Check sheet for the modelled part. Datum: model origin and axes. Units: mm. A direction names the side the tool comes from. Round coordinates to 2 decimals unless told otherwise and drop trailing zeros. Loops run counter-clockwise (first coordinate to the right, second up) from the corner with the lowest first, then second, coordinate; pieces in that order, holes last. Notation, with made-up numbers: M 77.5,24.25 L 124.5,24.25 A26 cw 124.5,51.25 Z; hole C 24.5,72 d11. An arc over 180 degrees is marked long. Write item = value, one per line. Start each with the question number.
(1) Cross-section at B-B on x = -24.5. Record the boundary of the cut face in (y, z).
(2) Cross-section at C-C on x = 7. Record the boundary of the cut face in (y, z), plus the area to 3 significant figures.
(3) Set-up check for faces 1 (the face through (-20, 12, 0)), 2 (the face through (20, 32, 0)), 3 (the face through (20, 12, 0)), 4 (the face through (-20, 30, 0)): record each of +Z, -Z, +X, -X, +Y, -Y from which the full face is reachable in a straight line by a thin tool's end or side.
(4) Mould release check, pull along X, two halves, no side actions. Record for faces 5 (the face through (0, 0, 0)), 6 (the face through (7, 37.5, 0)), 7 (the face through (-12.112, 35.472, -0.14)): pulls with the +X half, pulls with the -X half, needs draft (parallel to the pull), parting line crosses it, or undercut.
(5) Cross-section at D-D on z = 0. Record the boundary of the cut face in (x, y).
(6) Go/stop test with flat-tipped pins: P1, Ø9, axis at x = 25.5, z = 1, coming from the -Y side; P2, Ø10, axis at y = 13, z = -7, coming from the +X side; P3, Ø2.5, axis at x = -24.5, z = -1, coming from the +Y side. Record where each tip stops, or that it passes through.
(7) Cross-section at A-A on z = 5. Record the boundary of the cut face in (x, y), plus the area to 3 significant figures.
(8) Scan lines: L1, parallel to Z at x = 24.5, y = 26.6; L2, parallel to X at y = 26.2, z = 5; L3, parallel to Z at x = 7, y = 38. Record each from-to range of solid material in increasing order. Write a range as from..to.
Autodesk Inventor part; units mm, degrees
ref_plane "Work Plane1" through (0, 24.7, 0) normal (0, -1, 0) x (1, 0, 0)
ref_plane "YZ Plane" through (0, 0, 0) normal (1, 0, 0) x (0, 1, 0)
ref_plane "XZ Plane" through (0, 0, 0) normal (0, 1, 0) x (-1, 0, 0)
sketch "Sketch1" plane through (0, 0, 0) normal (0, 1, 0) x (-1, 0, 0)
  line L0 (20, 10) -> (-20, 10)
  line L1 (-20, 10) -> (-20, -10)
  line L2 (-20, -10) -> (20, -10)
  line L3 (20, -10) -> (20, 10)
  line L4 (20, 10) -> (-20, -10) construction
  line L5 (-20, 10) -> (20, -10) construction
  point P0 (0, 0)
  dimension "d0" = 40
  dimension "d1" = 20
extrude "Extrusion1" add sketch "Sketch1" along normal blind 37.5
ref_plane "Work Plane1" through (0, 24.7, 0) normal (0, -1, 0) x (1, 0, 0)
sketch "Sketch2" plane through (0, 24.7, 0) normal (0, -1, 0) x (1, 0, 0)
  line L0 (-28, 10) -> (28, 10)
  line L1 (28, 10) -> (28, -10)
  line L2 (28, -10) -> (-28, -10)
  line L3 (-28, -10) -> (-28, 10)
  line L4 (-28, 10) -> (28, -10) construction
  line L5 (28, 10) -> (-28, -10) construction
  point P0 (0, 0)
  dimension "d5" = 56
  dimension "d6" = 20
extrude "Extrusion2" add sketch "Sketch2" against normal blind 2.7
sketch "Sketch3" plane through (0, 27.4, 0) normal (0, 1, 0) x (1, 0, 0)
  circle A0 centre (-24.5, -5) radius 2
  line L0 (-28, 10) -> (-28, -10) construction
  line L1 (-28, 0) -> (28, 0) construction
  line L2 (28, 10) -> (28, -10) construction
  line L3 (-20, -10) -> (20, -10)
  line L4 (0, -10) -> (0, 10) construction
  line L5 (20, 10) -> (-20, 10)
  circle A1 centre (-24.5, 5) radius 2
  circle A2 centre (24.5, -5) radius 2
  circle A3 centre (24.5, 5) radius 2
  point P0 (0, 0)
  dimension "d9" = 4
  dimension "d10" = 5
  dimension "d11" = 24.5
extrude "Extrusion3" cut sketch "Sketch3" against normal up to surface (2.7 mm away)
sketch "Sketch4" plane through (0, 37.5, 0) normal (0, 1, 0) x (1, 0, 0)
  circle A0 centre (7, 0) radius 3
  line L0 (20, -10) -> (20, 10)
  point P0 (0, 0)
  dimension "d14" = 6
  dimension "d15" = 13
extrude "Extrusion4" add sketch "Sketch4" along normal blind 4
fillet "Fillet1" radius 2 4 edges at (-28, 26.05, 10) (28, 26.05, 10) (28, 26.05, -10) (-28, 26.05, -10)
chamfer "Chamfer1" distance 16 distance2 4 1 edges at (-20, 37.5, 0) measured on face at (-12, 37.5, 0)
sketch "Sketch5" plane through (7, 41.5, 0) normal (0, 1, 0) x (1, 0, 0)
  circle A0 centre (0, 0) radius 1.5
  circle A1 centre (0, 0) radius 3 construction
  point P0 (-7, 0)
  dimension "d22" = 3
extrude "Extrusion5" cut sketch "Sketch5" against normal blind 4
chamfer "Chamfer2" distance 0.25 angle 45 1 edges at (4, 41.5, 0)
properties part number "INJORA 35KG Digital Servo"
Result:
q1.outline = M 24.7,-10 L 27.4,-10 L 27.4,-7 L 24.7,-7 Z; M 24.7,-3 L 27.4,-3 L 27.4,3 L 24.7,3 Z; M 24.7,7 L 27.4,7 L 27.4,10 L 24.7,10 Z
q2.outline = M 0,-10 L 37.5,-10 L 37.5,-3 L 41.25,-3 L 41.5,-2.75 L 41.5,-1.5 L 37.5,-1.5 L 37.5,1.5 L 41.5,1.5 L 41.5,2.75 L 41.25,3 L 37.5,3 L 37.5,10 L 0,10 Z
q2.area = 762 mm^2
q3.face_1 = +Z, -Z, -X, -Y
q3.face_2 = +Z, -Z, +X, +Y
q3.face_3 = +Z, -Z, +X, -Y
q3.face_4 = +Z, -Z, -X, +Y
q4.face_5 = needs draft
q4.face_6 = undercut
q4.face_7 = pulls with the -X half
q5.outline = M -28,24.7 L -20,24.7 L -20,0 L 20,0 L 20,24.7 L 28,24.7 L 28,27.4 L 20,27.4 L 20,37.5 L 10,37.5 L 10,41.25 L 9.75,41.5 L 8.5,41.5 L 8.5,37.5 L 5.5,37.5 L 5.5,41.5 L 4.25,41.5 L 4,41.25 L 4,37.5 L -4,37.5 L -20,33.5 L -20,27.4 L -28,27.4 Z
q6.P1 = 24.7
q6.P2 = 20
q6.P3 = 27.4
q7.outline = M -28,24.7 L -26.5,24.7 L -26.5,27.4 L -28,27.4 Z; M -22.5,24.7 L -20,24.7 L -20,0 L 20,0 L 20,24.7 L 22.5,24.7 L 22.5,27.4 L 20,27.4 L 20,37.5 L -4,37.5 L -20,33.5 L -20,27.4 L -22.5,27.4 Z; M 26.5,24.7 L 28,24.7 L 28,27.4 L 26.5,27.4 Z
q7.area = 1,490 mm^2
q8.L1 = -10..-7, -3..3, 7..10
q8.L2 = -28..-26.5, -22.5..22.5, 26.5..28
q8.L3 = -3..-1.5, 1.5..3
